Part model, mm, in its own coordinate system. A direction names the side the tool comes from. Give positions to 0.01 mm unless a question says otherwise; leave off trailing zeros. Order: outer loops, then holes, each group sorted by start corner. A loop starts at its lowest first (then second) coordinate and runs counter-clockwise, first axis right, second up. Notation, with made-up numbers: (80.5, -5) - (102.5, -5) arc R21 cw to (102.5, 20) - close; hole circle Ø10 at (84, 64.5). An arc over 180 degrees is marked (long way). Use a Markdown table: item, result. Add a question column.
from build123d import *

# Parameters (mm, degrees)
F1_DEPTH = 33.02
F2_R     = 2.5273
F3_DEPTH = 25.4
F4_R     = 2.667
F5_DEPTH = 10.16


with BuildPart() as f1:
    # F0 (on Top) → F1 (new body)
    with BuildSketch(Plane.XY):
        with BuildLine():
            Line((7.099516, 6.35), (-7.099516, 6.35))
            ThreePointArc((-7.099516, 6.35), (0, -9.525), (7.099516, 6.35))
        make_face()
    extrude(amount=F1_DEPTH)

    # F2 (on face) → F3 (cut)
    with BuildSketch(Plane(origin=(0, 6.35, 0), x_dir=(-1, 0, 0), z_dir=(0, 1, 0))):
        with Locations((0, 7.62)):
            Circle(F2_R)
    extrude(amount=-F3_DEPTH, mode=Mode.SUBTRACT)

    # F4 (on face) → F5 (cut)
    with BuildSketch(Plane(origin=(0, 0, 0), x_dir=(1, 0, 0), z_dir=(0, 0, -1))):
        Circle(F4_R)
    extrude(amount=-F5_DEPTH, mode=Mode.SUBTRACT)


solid = f1.part
1. Mould opens along X. For faces 1 (the face through (-0.31, -9.52, 16.28)), 2 (the face through (1.231, 2.366, 3.88)), 3 (the face through (0, -3, 0)) say: released by +X, released by -X, zero draft, split by the parting line, or undercut.
2. Cut at C-C (z = 31). Write the cut outline in (x, y) (3 decimals), plus the area to 3 significant figures.
3. Cut at D-D (y = -4.75). Write the cut outline in (x, z).
4. Cut at A-A (x = 0). Write the cut outline in (y, z) (3 decimals).
5. Drill centre lines: probe 1 along Z at (x, y) = (0, 4.2); probe 2 along X at (y, z) = (2.7, 7.62); probe 3 along Y at (x, z) = (0, 2) (3 decimals). Where is each one in solid material? Low to high. Write a range as [from, to].
6. Cut at B-B (y = 0). Write the cut outline in (x, z) (3 decimals), plus the area to 3 significant figures.
7. Pin check, flat tips, straight feed: P1, Ø5, axis at y = 4.5, z = 3.5, coming from the -X side; P2, Ø4, axis at x = -3, z = 29, coming from the -Y side; P3, Ø3, axis at x = 0, z = 7.62, coming from the +Y side. Stop position of each tip, or through.
8. Tool access for faces 4 (the face through (0, 0, 10.16)), 5 (the face through (0, -1, 33.02)): list every direction of +Z, -Z, +X, -X, +Y, -Y with a clear straight run to the whole face (end or side of a thin tool).
Responses:
| question | item | result |
|---|---|---|
| 1 | face 1 | split by the parting line |
| 1 | face 2 | undercut |
| 1 | face 3 | zero draft |
| 2 | outline | (-7.1, 6.35) arc R9.525 ccw (long way) to (7.1, 6.35) - close |
| 2 | area | 254 mm² |
| 3 | outline | (-8.26, 0) - (8.26, 0) - (8.26, 33.02) - (-8.26, 33.02) - close; hole circle Ø5.05 at (0, 7.62) |
| 4 | outline | (-9.525, 0) - (-2.667, 0) - (-2.667, 5.093) - (-9.525, 5.093) - close; (-9.525, 10.147) - (-2.667, 10.147) - (-2.667, 10.16) - (2.667, 10.16) - (2.667, 10.147) - (6.35, 10.147) - (6.35, 33.02) - (-9.525, 33.02) - close; (2.667, 0) - (6.35, 0) - (6.35, 5.093) - (2.667, 5.093) - close |
| 5 | probe 1 | z = [0, 5.09], [10.15, 33.02] |
| 5 | probe 2 | x = [-9.13, -2.53], [2.53, 9.13] |
| 5 | probe 3 | y = [-9.525, -2.667], [2.667, 6.35] |
| 6 | outline | (-9.525, 0) - (-2.667, 0) - (-2.667, 10.16) - (2.667, 10.16) - (2.667, 0) - (9.525, 0) - (9.525, 33.02) - (-9.525, 33.02) - close |
| 6 | area | 575 mm² |
| 7 | P1 | stops at x = -9.31 |
| 7 | P2 | stops at y = -9.47 |
| 7 | P3 | passes through |
| 8 | face 4 | -Z |
| 8 | face 5 | +Z, +X, -X, +Y, -Y |
